Build history of the part. All positions in model axes, mm. A direction names the side the tool comes from. Coordinates: 2 decimals unless noted, no trailing zeros. Loops run counter-clockwise (first coordinate to the right, second up) from the corner with the lowest first, then second, coordinate; pieces in that order, holes last.
(1) Two-plate mould, pull along Y, no slides. Class faces 1 (the face through (20, 3, 34.999)), 2 (the face through (26.445, 23, 2)), 3 (the face through (11, 0, 20)), 4 (the face through (14.445, 22, 2)): pulls with the +Y half, pulls with the -Y half, needs draft (parallel to the pull), parting line crosses it, or undercut.
(2) Slice it at C-C (y = 16). Give the cut face in (x, z), and give its area (3 significant figures).
(3) Slice it at A-A (x = 24.5). Give the cut face in (y, z), and give its area (3 significant figures).
(4) Flat gauge pins, fed straight in: P1, Ø10, axis at x = 23.5, z = 18, coming from the +Y side; P2, Ø10, axis at x = 20, y = 31, coming from the +Z side. Where does each tip first touch, or does it go through?
(5) Slice it at B-B (z = 33). Give the cut face in (x, y), and give its area (3 significant figures).
(6) Wall check: L1, parallel to X at y = 13, z = 2; L2, parallel to Y at x = 6, z = 19. Give the ranges that are in metal, low to high.
(7) Tool access for faces 5 (the face through (20, 34.426, 2)), 6 (the face through (25.894, 3, 23)), 7 (the face through (11, 5, 23)): list every direction of +Z, -Z, +X, -X, +Y, -Y with a clear straight run to the whole face (end or side of a thin tool).
(8) Slice it at D-D (y = 3). Give the cut face in (x, z), and give its area (3 significant figures).
Autodesk Fusion 360 part; units mm, degrees
sketch "Esquisse1" plane through (0, 0, 0) normal (1, 0, 0) x (0, 1, 0)
  line L0 (0, 0) -> (40, 0)
  line L1 (0, 0) -> (0, 40)
  line L2 (0, 40) -> (5, 40)
  line L3 (5, 40) -> (5, 5)
  line L4 (5, 5) -> (40, 5)
  line L5 (40, 5) -> (40, 0)
  dimension "d2" = 40
extrude "Extrusion1" add sketch "Esquisse1" along normal blind 30
sketch "Esquisse2" plane through (0, 0, 0) normal (0, 0, 1) x (1, 0, 0)
  line L0 (9.4451, 34.4261) -> (21.4451, 34.4261)
  line L1 (21.4451, 34.4261) -> (21.4451, 10.4261)
  line L2 (21.4451, 10.4261) -> (9.4451, 10.4261)
  line L3 (9.4451, 10.4261) -> (9.4451, 34.4261)
  dimension "d5" = 12
  dimension "d6" = 24
extrude "Extrusion2" cut sketch "Esquisse2" along normal blind 6
sketch "Esquisse4" plane through (0, 5, 0) normal (0, 1, 0) x (-1, 0, 0)
  line L0 (0, 5) -> (0, 40)
  line L1 (0, 40) -> (-30, 40)
  line L2 (-30, 40) -> (-30, 5)
  line L3 (-30, 5) -> (0, 5)
  line L4 (-8.8938, 10.999) -> (-20.8938, 10.999)
  line L5 (-20.8938, 10.999) -> (-20.8938, 34.999)
  line L6 (-20.8938, 34.999) -> (-8.8938, 34.999)
  line L7 (-8.8938, 34.999) -> (-8.8938, 10.999)
  dimension "d15" = 12
  dimension "d16" = 24
extrude "Extrusion3" cut sketch "Esquisse4" against normal blind 34 contours L4 L5 L6 L7
extrude "Extrusion4" cut 1 faces at (20.8938, 3.3333, 18.999) along direction (1, 0, 0) blind 5
extrude "Extrusion5" add 1 faces at (8.8938, 3.3333, 26.999) along direction (1, 0, 0) blind 5
extrude "Extrusion6" cut 1 faces at (21.4451, 26.4261, 1.6667) along direction (1, 0, 0) blind 5
extrude "Extrusion7" add 1 faces at (9.4451, 18.4261, 1.6667) along direction (1, 0, 0) blind 5
Response values:
1. face 1: needs draft
1. face 2: undercut
1. face 3: pulls with the -Y half
1. face 4: undercut
2. outline: (0, 0) - (14.45, 0) - (14.45, 5) - (0, 5) - close; (26.45, 0) - (30, 0) - (30, 5) - (26.45, 5) - close
2. area: 90.0 mm2
3. outline: (0, 0) - (10.43, 0) - (10.43, 5) - (5, 5) - (5, 11) - (0, 11) - close; (0, 35) - (5, 35) - (5, 40) - (0, 40) - close; (34.43, 0) - (40, 0) - (40, 5) - (34.43, 5) - close
3. area: 135 mm2
4. P1: stops at y = 5
4. P2: stops at z = 5
5. outline: (0, 0) - (13.89, 0) - (13.89, 5) - (0, 5) - close; (25.89, 0) - (30, 0) - (30, 5) - (25.89, 5) - close
5. area: 90.0 mm2
6. L1: x = 0 to 14.45, 26.45 to 30
6. L2: y = 0 to 5
7. face 5: +Z, -Z
7. face 6: +Y, -Y
7. face 7: +Z, +X, -X, +Y
8. outline: (0, 0) - (30, 0) - (30, 40) - (0, 40) - close; hole (13.89, 11) - (25.89, 11) - (25.89, 35) - (13.89, 35) - close
8. area: 912 mm2
